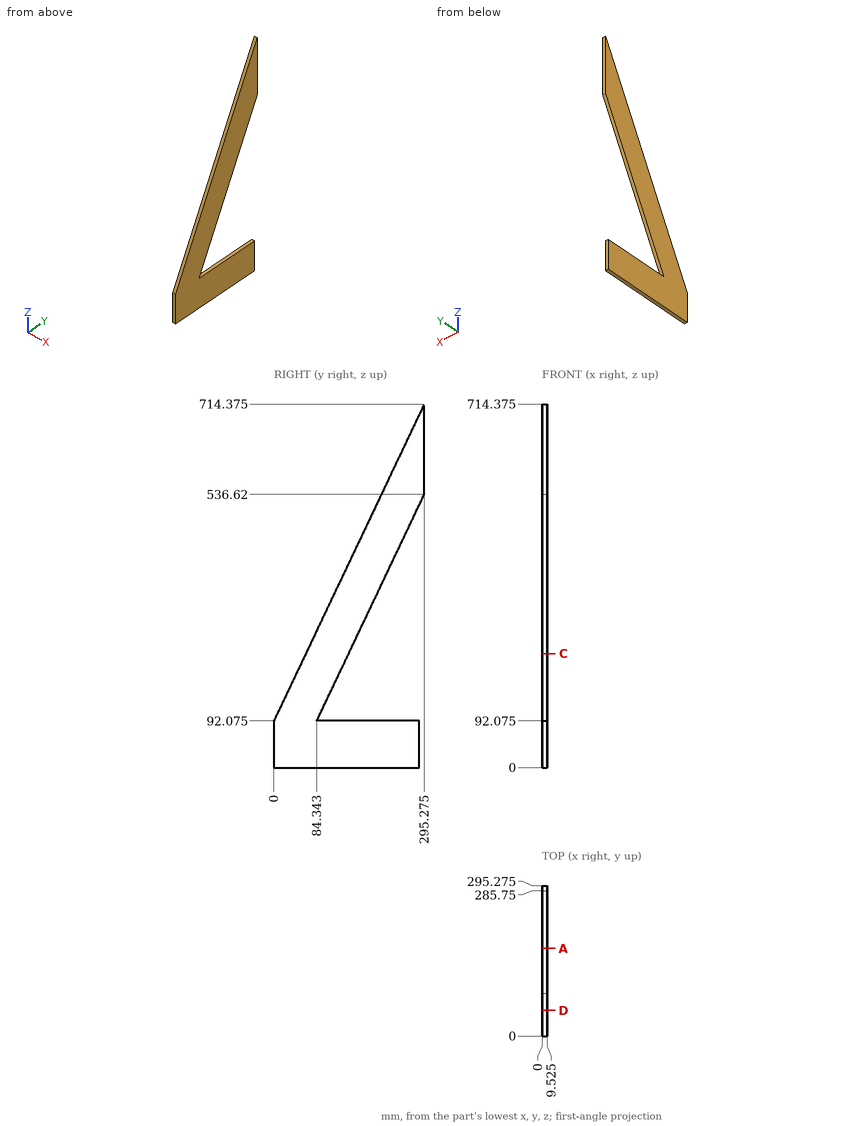
Study the drawing (mm; zero at the part's minimum x, y, z) and answer. Coordinates: 2 decimals unless noted, no trailing zeros. Loops run counter-clockwise (first coordinate to the right, second up) from the corner with the lowest first, then second, coordinate; pieces in that order, holes last. Notation, with made-up numbers: (-10, -20.75) -> (3, -20.75) arc R11 ccw to (3, -8.75) -> close; hole circle Ø3 at (-6.75, -35). An arc over 180 degrees is marked (long way). Answer in a Markdown table with one row per item. Add a question column.
1. Consider line 1 (Z direction, x = 2.75, y = 274) (1 decimal); line 2 (Z direction, x = 7.5, y = 275.5) (1 decimal); line 3 (Y direction, x = 6.25, z = 127) (1 decimal). Determine where each line is inside the solid, lowest interval first. Write a range as [from, to].
2. The part is cut by section A-A, the plane y = 172. Write down the section's boundary in (x, z) (1 decimal).
3. Flat-ended cylindrical pins translate along their axes: P1, Ø4, axis at y = 99, z = 307.5, coming from the -X side; P2, Ø5, axis at x = 5, z = 440, coming from the -Y side; P3, Ø1, axis at x = 7.5, y = 241.5, coming from the +Z side (1 decimal); P4, Ø1, axis at x = 6, z = 284, coming from the +Y side. Find the tip coordinate at first contact, or state that the pin passes through.
4. The part is cut by section D-D, the plane y = 50.5. Write down the section's boundary in (x, z) (1 decimal), then the cut area to 3 significant figures.
5. The part is cut by section C-C, the plane z = 224. Write down the section's boundary in (x, y) (1 decimal), then the cut area to 3 significant figures.
Answer below:
| question | item | result |
|---|---|---|
| 1 | line 1 | [0, 92.1], [491.8, 669.5] |
| 1 | line 2 | [0, 92.1], [494.9, 672.7] |
| 1 | line 3 | [16.6, 100.9] |
| 2 | outline | (0, 0) -> (9.5, 0) -> (9.5, 92.1) -> (0, 92.1) -> close; (0, 276.8) -> (9.5, 276.8) -> (9.5, 454.6) -> (0, 454.6) -> close |
| 3 | P1 | through |
| 3 | P2 | y = 163.9 |
| 3 | P3 | z = 602.1 |
| 3 | P4 | y = 175.65 |
| 4 | outline | (0, 0) -> (9.5, 0) -> (9.5, 198.5) -> (0, 198.5) -> close |
| 4 | area | 1,890 mm2 |
| 5 | outline | (0, 62.6) -> (9.5, 62.6) -> (9.5, 146.9) -> (0, 146.9) -> close |
| 5 | area | 803 mm2 |
